Design review of the part built by this model. Coordinates are the model's own, in mm. A direction names the side the tool comes from. Give positions to 0.01 mm unless a question says otherwise; leave off trailing zeros. Loops run counter-clockwise (first coordinate to the right, second up) from the corner with the lowest first, then second, coordinate; pieces in that order, holes last. Notation, with made-up numbers: (86.25, 54) - (103.25, 54) arc R31 cw to (103.25, 80) - close; hole circle Ø6 at (41.25, -36). An arc over 180 degrees is marked (long way). Write each question's results on one line, items separated by ' | '.
```python
from build123d import *

# Parameters (mm, degrees)
SKETCH2_W               = 42
SKETCH2_H               = 17.8
BOSS_EXTRUDE1_DEPTH     = 4
SKETCH3_W               = 2
SKETCH3_H               = 17.8
BOSS_EXTRUDE2_DEPTH     = 10
BOSS_EXTRUDE3_DEPTH     = 2
SKETCH5_R               = 2.5
CUT_EXTRUDE1_DEPTH      = 11
CUT_EXTRUDE1_DEPTH_BACK = 5
SKETCH6_R               = 1.25
CUT_EXTRUDE2_DEPTH      = 2
SKETCH7_W               = 2
SKETCH7_H               = 17.8
BOSS_EXTRUDE4_DEPTH     = 10
SKETCH8_R               = 1.25
CUT_EXTRUDE3_DEPTH      = 10
BOSS_EXTRUDE5_DEPTH     = 2


with BuildPart() as part:
    # Sketch2 → Boss-Extrude1 (new body)
    with BuildSketch(Plane(origin=(0, 0, 0), x_dir=(1, 0, 0), z_dir=(0, 1, 0))):
        Rectangle(SKETCH2_W, SKETCH2_H)
    extrude(amount=BOSS_EXTRUDE1_DEPTH)

    # Sketch3 → Boss-Extrude2 (add)
    with BuildSketch(Plane.XZ):
        with Locations((-20, 0)):
            Rectangle(SKETCH3_W, SKETCH3_H)
        with Locations((20, 0)):
            Rectangle(SKETCH3_W, SKETCH3_H)
    extrude(amount=BOSS_EXTRUDE2_DEPTH)

    # Sketch4 → Boss-Extrude3 (add)
    with BuildSketch(Plane.XY.offset(8.9)):
        Polygon((-19, 0), (-14, 0), (-19, -5), align=None)
        Polygon((19, -5), (14, 0), (19, 0), align=None)
    boss_extrude3 = extrude(amount=-BOSS_EXTRUDE3_DEPTH)

    # Mirror1: Boss-Extrude3 across plane
    add(boss_extrude3.mirror(Plane.XY))

    # Sketch5 → Cut-Extrude1 (cut, two sides)
    with BuildSketch(Plane.XZ) as cut_extrude1_sk:
        with Locations((-8.319906625, 0)):
            Circle(SKETCH5_R)
        with Locations((6.680093375, 0)):
            Circle(SKETCH5_R)
    extrude(amount=CUT_EXTRUDE1_DEPTH, mode=Mode.SUBTRACT)
    extrude(cut_extrude1_sk.sketch, amount=-CUT_EXTRUDE1_DEPTH_BACK, mode=Mode.SUBTRACT)

    # Sketch6 → Cut-Extrude2 (cut)
    with BuildSketch(Plane(origin=(-19, 0, 0), x_dir=(0, 0, -1), z_dir=(1, 0, 0))):
        with Locations((-4, -3)):
            Circle(SKETCH6_R)
        with Locations((4, -3)):
            Circle(SKETCH6_R)
    cut_extrude2 = extrude(amount=-CUT_EXTRUDE2_DEPTH, mode=Mode.SUBTRACT)

    # Mirror2: Cut-Extrude2 across plane
    add(cut_extrude2.mirror(Plane(origin=(0, 0, 0), x_dir=(0, 0, 1), z_dir=(1, 0, 0))), mode=Mode.SUBTRACT)

    # Sketch7 → Boss-Extrude4 (add)
    with BuildSketch(Plane(origin=(0, 4, 0), x_dir=(1, 0, 0), z_dir=(0, 1, 0))):
        with Locations((-20, 0)):
            Rectangle(SKETCH7_W, SKETCH7_H)
        with Locations((20, 0)):
            Rectangle(SKETCH7_W, SKETCH7_H)
    extrude(amount=BOSS_EXTRUDE4_DEPTH)

    # Sketch8 → Cut-Extrude3 (cut)
    with BuildSketch(Plane(origin=(-19, 0, 0), x_dir=(0, 0, -1), z_dir=(1, 0, 0))):
        with Locations((-4, 7)):
            Circle(SKETCH8_R)
        with Locations((4, 7)):
            Circle(SKETCH8_R)
    cut_extrude3 = extrude(amount=-CUT_EXTRUDE3_DEPTH, mode=Mode.SUBTRACT)

    # Mirror3: Cut-Extrude3 across plane
    add(cut_extrude3.mirror(Plane(origin=(0, 0, 0), x_dir=(0, 0, 1), z_dir=(1, 0, 0))), mode=Mode.SUBTRACT)

    # Sketch9 → Boss-Extrude5 (add)
    with BuildSketch(Plane(origin=(0, 0, -8.9), x_dir=(-1, 0, 0), z_dir=(0, 0, -1))):
        Polygon((-19, 9), (-19, 4), (-14, 4), align=None)
        Polygon((19, 9), (14, 4), (19, 4), align=None)
    boss_extrude5 = extrude(amount=-BOSS_EXTRUDE5_DEPTH)

    # Mirror4: Boss-Extrude5 across plane
    add(boss_extrude5.mirror(Plane.XY))


solid = part.part
```
Item 1: We need section C-C on y = 7. Give the number of separate pieces and of enclosed holes in the cut face, then the cut area to 3 significant figures.
Output values:
separate pieces: 6 | enclosed holes: 0 | area: 67.2 mm²
Item 2: We need section D-D on x = 18. Give the boundary of the cut face in (y, z).
Output values:
outline: (-4, -8.9) - (8, -8.9) - (8, -6.9) - (4, -6.9) - (4, 6.9) - (8, 6.9) - (8, 8.9) - (-4, 8.9) - (-4, 6.9) - (0, 6.9) - (0, -6.9) - (-4, -6.9) - close
Item 3: Clearance check with flat-ended pins moving along their axes: P1, Ø4, axis at y = 7, z = 4, coming from the -X side; P2, Ø9, axis at x = 4.5, z = -1.5, coming from the +Y side; P3, Ø6, axis at x = -6.5, z = 6.5, coming from the -Y side. State where each tip first meets the part, or that it passes through.
Output values:
P1: stops at x = -21 | P2: stops at y = 4 | P3: stops at y = 0
Item 4: We need section B-B on y = -8. Give the boundary of the cut face in (x, z), then the cut area to 3 significant figures.
Output values:
outline: (-21, -8.9) - (-19, -8.9) - (-19, 8.9) - (-21, 8.9) - close; (19, -8.9) - (21, -8.9) - (21, 8.9) - (19, 8.9) - close | area: 71.2 mm²
Item 5: We need section A-A on z = 0. Give the boundary of the cut face in (x, y), then the cut area to 3 significant figures.
Output values:
outline: (-21, -10) - (-19, -10) - (-19, 0) - (-10.82, 0) - (-10.82, 4) - (-19, 4) - (-19, 14) - (-21, 14) - close; (-5.82, 0) - (4.18, 0) - (4.18, 4) - (-5.82, 4) - close; (9.18, 0) - (19, 0) - (19, -10) - (21, -10) - (21, 14) - (19, 14) - (19, 4) - (9.18, 4) - close | area: 208 mm²
Item 6: Wall thickness on probe 1 along Y at (x, z) = (-20.4, 4); probe 2 along X at (y, z) = (12.75, -5); probe 3 along Z at (x, y) = (20.35, 7): over which ranges is each line inside the solid? List them lowest first.
Output values:
probe 1: y = -10 to -4.25, -1.75 to 5.75, 8.25 to 14 | probe 2: x = -21 to -19, 19 to 21 | probe 3: z = -8.9 to -5.25, -2.75 to 2.75, 5.25 to 8.9
Item 7: Tool access review of faces 4 (the face through (19, 9, 0)), 5 (the face through (19, -5, 0)), 6 (the face through (-16, -2, 8)): name each direction out of +Z, -Z, +X, -X, +Y, -Y from which nothing blocks a thin tool from reaching the whole face with its end or side.
Output values:
face 4: +Y | face 5: -Y | face 6: +Z, -Z, -Y
Item 8: Draft analysis for pull direction X (two halves, no side actions). For faces 1 (the face through (-19.986, -2.155, 4.921)), 2 (the face through (-18, 5, 6.9)), 3 (the face through (-21, 2, 0)), state which applies: +X half, -X half, draft (parallel to the pull), parting line (faces both ways), or undercut.
Output values:
face 1: draft | face 2: undercut | face 3: -X half
